Geometry: final body of the model. Coordinates: model frame, mm. A direction names the side the tool comes from. Give positions to 0.01 mm unless a question says otherwise; leave off trailing zeros. Loops run counter-clockwise (first coordinate to the right, second up) from the corner with the lowest first, then second, coordinate; pieces in that order, holes last.
from build123d import *

# Parameters (mm, degrees)
ESQUISSE1_W             = 71
ESQUISSE1_H             = 24.2
BOSS_EXTRU_1_DEPTH      = 9
ENL_V_MAT_EXTRU_1_DEPTH = 1
ENL_V_MAT_EXTRU_2_DEPTH = 1
ESQUISSE4_W             = 22
ESQUISSE4_H             = 4
ESQUISSE4_W_2           = 4
ENL_V_MAT_EXTRU_3_DEPTH = 0.2
ESQUISSE5_W             = 4
ESQUISSE5_H             = 1
ESQUISSE5_H_2           = 18
ENL_V_MAT_EXTRU_4_DEPTH = 0.2


with BuildPart() as part:
    # Esquisse1 → Boss.-Extru.1 (new body)
    with BuildSketch(Plane.XY):
        Rectangle(ESQUISSE1_W, ESQUISSE1_H)
    extrude(amount=BOSS_EXTRU_1_DEPTH)

    # Esquisse2 → Enlèv. mat.-Extru.1 (cut)
    with BuildSketch(Plane.XY.offset(9)):
        with BuildLine():
            Line((-31.25, 7.1), (31.25, 7.1))
            ThreePointArc((31.25, 7.1), (31.957106781, 6.807106781), (32.25, 6.1))
            Line((32.25, 6.1), (32.25, -6.1))
            ThreePointArc((32.25, -6.1), (31.957106781, -6.807106781), (31.25, -7.1))
            Line((31.25, -7.1), (-31.25, -7.1))
            ThreePointArc((-31.25, -7.1), (-31.957106781, -6.807106781), (-32.25, -6.1))
            Line((-32.25, -6.1), (-32.25, 6.1))
            ThreePointArc((-32.25, 6.1), (-31.957106781, 6.807106781), (-31.25, 7.1))
        make_face()
    extrude(amount=-ENL_V_MAT_EXTRU_1_DEPTH, mode=Mode.SUBTRACT)

    # Esquisse3 → Enlèv. mat.-Extru.2 (cut)
    with BuildSketch(Plane.XY.offset(9)):
        with BuildLine():
            Line((-32.25, 10.5), (32.25, 10.5))
            ThreePointArc((32.25, 10.5), (32.75, 10), (32.25, 9.5))
            Line((32.25, 9.5), (-32.25, 9.5))
            ThreePointArc((-32.25, 9.5), (-32.75, 10), (-32.25, 10.5))
        make_face()
        with BuildLine():
            Line((-32.25, -10.5), (32.25, -10.5))
            ThreePointArc((32.25, -10.5), (32.75, -10), (32.25, -9.5))
            Line((32.25, -9.5), (-32.25, -9.5))
            ThreePointArc((-32.25, -9.5), (-32.75, -10), (-32.25, -10.5))
        make_face()
    extrude(amount=-ENL_V_MAT_EXTRU_2_DEPTH, mode=Mode.SUBTRACT)

    # Esquisse4 → Enlèv. mat.-Extru.3 (cut)
    with BuildSketch(Plane.XZ.offset(12.1)):
        with Locations((14.5, 0)):
            Rectangle(ESQUISSE4_W, ESQUISSE4_H)
        with Locations((-14.5, 0)):
            Rectangle(ESQUISSE4_W, ESQUISSE4_H)
        with Locations((35.5, 0)):
            Rectangle(ESQUISSE4_W_2, ESQUISSE4_H)
        with Locations((-35.5, 0)):
            Rectangle(ESQUISSE4_W_2, ESQUISSE4_H)
    enl_v_mat_extru_3 = extrude(amount=-ENL_V_MAT_EXTRU_3_DEPTH, mode=Mode.SUBTRACT)

    # Symétrie1: Enlèv. mat.-Extru.3 across plane
    add(enl_v_mat_extru_3.mirror(Plane.ZX), mode=Mode.SUBTRACT)

    # Esquisse5 → Enlèv. mat.-Extru.4 (cut)
    with BuildSketch(Plane(origin=(35.5, 0, 0), x_dir=(0, 0, -1), z_dir=(1, 0, 0))):
        with Locations((0, 11.6)):
            Rectangle(ESQUISSE5_W, ESQUISSE5_H)
        Rectangle(ESQUISSE5_W, ESQUISSE5_H_2)
        with Locations((0, -11.6)):
            Rectangle(ESQUISSE5_W, ESQUISSE5_H)
    enl_v_mat_extru_4 = extrude(amount=-ENL_V_MAT_EXTRU_4_DEPTH, mode=Mode.SUBTRACT)

    # Symétrie2: Enlèv. mat.-Extru.4 across plane
    add(enl_v_mat_extru_4.mirror(Plane(origin=(0, 0, 0), x_dir=(0, 0, 1), z_dir=(1, 0, 0))), mode=Mode.SUBTRACT)


solid = part.part
Item 1: Draft query along Y for faces 4 (the face through (35.5, 0, 5)), 5 (the face through (-35.3, 0, 1)), 6 (the face through (35.3, 0, 1)), 7 (the face through (-15, -11.9, 1)). Return one class per face: +Y half, -Y half, draft (parallel to the pull), parting line (faces both ways), or undercut.
Values follow:
face 4: draft
face 5: undercut
face 6: undercut
face 7: -Y half
Item 2: Section query B-B on y = 3. Return loops of the section in (x, z).
Values follow:
outline: (-35.5, 2) - (-35.3, 2) - (-35.3, 0) - (35.3, 0) - (35.3, 2) - (35.5, 2) - (35.5, 9) - (32.25, 9) - (32.25, 8) - (-32.25, 8) - (-32.25, 9) - (-35.5, 9) - close
Item 3: Pin query (flat end, axial travel): pin 1 (4 mm diameter, centred on x = 0, y = 5.5, fed in from -Z); pin 2 (0.6 mm diameter, centred on y = 11.5, z = 0.5, fed in from +X); pin 3 (0.6 mm diameter, centred on x = -19.5, z = 1, fed in from +Y); pin 4 (0.6 mm diameter, centred on y = -11.5, z = 1.5, fed in from -X). Return the tip coordinate at first contact, or that it passes through.
Values follow:
pin 1: stops at z = 0
pin 2: stops at x = 35.3
pin 3: stops at y = 11.9
pin 4: stops at x = -35.3
Item 4: Section query C-C on x = 9. Return loops of the section in (y, z), plus the area to 3 significant figures.
Values follow:
outline: (-12.1, 2) - (-11.9, 2) - (-11.9, 0) - (11.9, 0) - (11.9, 2) - (12.1, 2) - (12.1, 9) - (10.5, 9) - (10.5, 8) - (9.5, 8) - (9.5, 9) - (7.1, 9) - (7.1, 8) - (-7.1, 8) - (-7.1, 9) - (-9.5, 9) - (-9.5, 8) - (-10.5, 8) - (-10.5, 9) - (-12.1, 9) - close
area: 201 mm2
Item 5: Ray query, probe 1 along Z at (x, y) = (-10.5, 6); probe 2 along X at (y, z) = (7.75, 1.5); probe 3 along Y at (x, z) = (20, 1.75). Return the intervals inside material, ascending.
Values follow:
probe 1: z = 0 to 8
probe 2: x = -35.3 to 35.3
probe 3: y = -11.9 to 11.9
Item 6: Section query A-A on x = 27. Return loops of the section in (y, z).
Values follow:
outline: (-12.1, 0) - (12.1, 0) - (12.1, 9) - (10.5, 9) - (10.5, 8) - (9.5, 8) - (9.5, 9) - (7.1, 9) - (7.1, 8) - (-7.1, 8) - (-7.1, 9) - (-9.5, 9) - (-9.5, 8) - (-10.5, 8) - (-10.5, 9) - (-12.1, 9) - close
Item 7: Set-up query: faces 1 (the face through (14, 11.9, 1)), 2 (the face through (34, 11.9, 1)), 3 (the face through (-34, -11.9, 1)). Return all of +Z, -Z, +X, -X, +Y, -Y with unobstructed straight access to the full face (end or side cutting, diameter ignored); none if empty.
Values follow:
face 1: -Z, +Y
face 2: -Z, +X, +Y
face 3: -Z, -X, -Y
